Read the model definition and answer for the solid it produces. Units are mm, in the model's axes. A direction names the side the tool comes from. Give positions to 0.01 mm unless a question says otherwise; leave off trailing zeros. Write each loop counter-clockwise with the first axis right and the second up, starting at its lowest first coordinate (ties: lowest second). Pieces come first, ordered by that corner, then holes. Notation, with made-up numbers: (-1.5, 11) -> (53.5, 11) arc R18 ccw to (53.5, 27) -> close; hole circle Ø5 at (0, 32). An arc over 180 degrees is marked (long way). Use a Markdown table: item, result.
from build123d import *
from OCP.BRepFilletAPI import BRepFilletAPI_MakeChamfer

# Parameters (mm, degrees)
SKETCH1_W                = 120
SKETCH1_H                = 70
BOSS_EXTRUDE1_DEPTH      = 5
SKETCH4_W                = 10
SKETCH4_H                = 10
BOSS_EXTRUDE2_DEPTH      = 30
SKETCH5_W                = 10
SKETCH5_H                = 5
CUT_EXTRUDE2_DEPTH       = 10
SKETCH8_W                = 10
SKETCH8_H                = 7
BOSS_EXTRUDE5_DEPTH      = 4
M3_CLEARANCE_HOLE2_D     = 3.4
M3_CLEARANCE_HOLE2_DEPTH = 65
M3_CLEARANCE_HOLE2_TIP   = 1.021463052
SKETCH12_W               = 65.5
SKETCH12_H               = 70
BOSS_EXTRUDE6_DEPTH      = 5
BOSS_EXTRUDE7_DEPTH      = 35
M3_CLEARANCE_HOLE3_D     = 3.4
M3_CLEARANCE_HOLE3_DEPTH = 65
M3_CLEARANCE_HOLE3_TIP   = 1.021463052
SKETCH24_W               = 10
SKETCH24_H               = 50
BOSS_EXTRUDE10_DEPTH     = 10
SKETCH16_W               = 10
SKETCH16_H               = 22
CUT_EXTRUDE5_DEPTH       = 133.665933834
SKETCH22_R               = 1.7
CUT_EXTRUDE7_DEPTH       = 20
CHAMFER2_SIZE            = 10
CHAMFER2_SIZE_2          = 14
SKETCH25_W               = 5.49
SKETCH25_H               = 3
CUT_EXTRUDE8_DEPTH       = 8
CUT_EXTRUDE9_START       = -20
SKETCH26_R               = 1.7
CUT_EXTRUDE9_DEPTH       = 20
CUT_EXTRUDE11_DEPTH      = 10
LPATTERN1_COUNT          = 2
LPATTERN1_PITCH          = 110
SKETCH29_W               = 10
SKETCH29_H               = 4.75
BOSS_EXTRUDE11_DEPTH     = 15
SKETCH31_R               = 1.7
CUT_EXTRUDE13_DEPTH      = 153.152062096


with BuildPart() as part:
    # Sketch1 → Boss-Extrude1 (new body)
    with BuildSketch(Plane(origin=(0, 0, 0), x_dir=(1, 0, 0), z_dir=(0, 1, 0))):
        Rectangle(SKETCH1_W, SKETCH1_H)
    extrude(amount=BOSS_EXTRUDE1_DEPTH)

    # Sketch4 → Boss-Extrude2 (add)
    with BuildSketch(Plane(origin=(0, 5, 0), x_dir=(1, 0, 0), z_dir=(0, 1, 0))):
        with Locations((-55, -30)):
            Rectangle(SKETCH4_W, SKETCH4_H)
        with Locations((-55, 30)):
            Rectangle(SKETCH4_W, SKETCH4_H)
        with Locations((55, -30)):
            Rectangle(SKETCH4_W, SKETCH4_H)
        with Locations((55, 30)):
            Rectangle(SKETCH4_W, SKETCH4_H)
    extrude(amount=BOSS_EXTRUDE2_DEPTH)

    # Sketch5 → Cut-Extrude2 (cut)
    with BuildSketch(Plane.XZ):
        with Locations((-55, -27.5)):
            Rectangle(SKETCH5_W, SKETCH5_H)
        with Locations((-55, 27.5)):
            Rectangle(SKETCH5_W, SKETCH5_H)
        with Locations((55, 27.5)):
            Rectangle(SKETCH5_W, SKETCH5_H)
        with Locations((55, -27.5)):
            Rectangle(SKETCH5_W, SKETCH5_H)
    extrude(amount=-CUT_EXTRUDE2_DEPTH, mode=Mode.SUBTRACT)

    # Sketch8 → Boss-Extrude5 (add)
    with BuildSketch(Plane(origin=(0, 5, 0), x_dir=(1, 0, 0), z_dir=(0, 1, 0))):
        with Locations((-45, 31.5)):
            Rectangle(SKETCH8_W, SKETCH8_H)
        with Locations((-45, -31.5)):
            Rectangle(SKETCH8_W, SKETCH8_H)
        with Locations((45, -31.5)):
            Rectangle(SKETCH8_W, SKETCH8_H)
        with Locations((45, 31.5)):
            Rectangle(SKETCH8_W, SKETCH8_H)
    extrude(amount=BOSS_EXTRUDE5_DEPTH)

    # M3 Clearance Hole2
    with Locations(Plane(origin=(0, 9, 0), x_dir=(1, 0, 0), z_dir=(0, 1, 0))):
        with Locations((-43.5, -31.5), (-43.5, 31.5), (43.5, 31.5), (43.5, -31.5)):
            Hole(M3_CLEARANCE_HOLE2_D / 2, depth=M3_CLEARANCE_HOLE2_DEPTH)
            with Locations((0, 0, -(M3_CLEARANCE_HOLE2_DEPTH + M3_CLEARANCE_HOLE2_TIP / 2))):  # 118° drill point
                Cone(0, M3_CLEARANCE_HOLE2_D / 2, M3_CLEARANCE_HOLE2_TIP, mode=Mode.SUBTRACT)

    # Sketch12 → Boss-Extrude6 (add)
    with BuildSketch(Plane.XZ):
        with Locations((92.75, 0)):
            Rectangle(SKETCH12_W, SKETCH12_H)
    extrude(amount=-BOSS_EXTRUDE6_DEPTH)

    # Sketch13 → Boss-Extrude7 (add)
    with BuildSketch(Plane(origin=(0, 5, 0), x_dir=(1, 0, 0), z_dir=(0, 1, 0))):
        Polygon((60, 35), (125.5, 35), (125.5, -35), (60, -35), (60, -30.5), (121, -30.5), (121, 30.5), (60, 30.5), align=None)
    extrude(amount=BOSS_EXTRUDE7_DEPTH)

    # M3 Clearance Hole3
    with Locations(Plane(origin=(0, 5, 0), x_dir=(1, 0, 0), z_dir=(0, 1, 0))):
        with Locations((117, -26.5), (117, 26.5), (64, 26.5), (64, -26.5)):
            Hole(M3_CLEARANCE_HOLE3_D / 2, depth=M3_CLEARANCE_HOLE3_DEPTH)
            with Locations((0, 0, -(M3_CLEARANCE_HOLE3_DEPTH + M3_CLEARANCE_HOLE3_TIP / 2))):  # 118° drill point
                Cone(0, M3_CLEARANCE_HOLE3_D / 2, M3_CLEARANCE_HOLE3_TIP, mode=Mode.SUBTRACT)

    # Sketch24 → Boss-Extrude10 (add)
    with BuildSketch(Plane(origin=(0, 5, 0), x_dir=(1, 0, 0), z_dir=(0, 1, 0))):
        with Locations((-55, 0)):
            Rectangle(SKETCH24_W, SKETCH24_H)
        with Locations((55, 0)):
            Rectangle(SKETCH24_W, SKETCH24_H)
    extrude(amount=BOSS_EXTRUDE10_DEPTH)

    # Sketch16 → Cut-Extrude5 (cut, through all)
    with BuildSketch(Plane(origin=(0, 15, 0), x_dir=(1, 0, 0), z_dir=(0, 1, 0))):
        with Locations((55, 0)):
            Rectangle(SKETCH16_W, SKETCH16_H)
    extrude(amount=-CUT_EXTRUDE5_DEPTH, mode=Mode.SUBTRACT)

    # Sketch22 → Cut-Extrude7 (cut)
    with BuildSketch(Plane.XY.offset(35)):
        with Locations((-55, 5)):
            Circle(SKETCH22_R)
        with Locations((55, 5)):
            Circle(SKETCH22_R)
    extrude(amount=-CUT_EXTRUDE7_DEPTH, mode=Mode.SUBTRACT)

    # Chamfer2
    chamfer2_edges_1 = [part.edges().sort_by_distance(p)[0] for p in [
        (55, 15, 11),
    ]]
    chamfer2_side_1 = [part.faces().sort_by_distance(p)[0] for p in [
        (55, 14.8, 11),
    ]]
    chamfer2_edges_2 = [part.edges().sort_by_distance(p)[0] for p in [
        (55, 15, -11),
    ]]
    chamfer2_side_2 = [part.faces().sort_by_distance(p)[0] for p in [
        (55, 14.8, -11),
    ]]
    chamfer2 = BRepFilletAPI_MakeChamfer(part.part.solid().wrapped)
    for e in chamfer2_edges_1:
        chamfer2.Add(CHAMFER2_SIZE - 0.0001, CHAMFER2_SIZE_2 - 0.0001, e.wrapped, chamfer2_side_1[0].wrapped)
    for e in chamfer2_edges_2:
        chamfer2.Add(CHAMFER2_SIZE - 0.0001, CHAMFER2_SIZE_2 - 0.0001, e.wrapped, chamfer2_side_2[0].wrapped)
    add(Compound.cast(chamfer2.Shape()), mode=Mode.REPLACE)  # a hair under: the kernel refuses the full size

    # Sketch25 → Cut-Extrude8 (cut)
    with BuildSketch(Plane.XZ):
        with Locations((-55, -18.5)):
            Rectangle(SKETCH25_W, SKETCH25_H)
        with Locations((55, -18.5)):
            Rectangle(SKETCH25_W, SKETCH25_H)
        with Locations((55, 18.5)):
            Rectangle(SKETCH25_W, SKETCH25_H)
        with Locations((-55, 18.5)):
            Rectangle(SKETCH25_W, SKETCH25_H)
    extrude(amount=-CUT_EXTRUDE8_DEPTH, mode=Mode.SUBTRACT)

    # Sketch26 → Cut-Extrude9 (cut)
    with BuildSketch(Plane(origin=(0, 0, -35), x_dir=(-1, 0, 0), z_dir=(0, 0, -1)).offset(CUT_EXTRUDE9_START)):
        with Locations(Location((-55, 5, 0), (0, 0, 180))):
            Circle(SKETCH26_R)
        with Locations(Location((55, 5, 0), (0, 0, 180))):
            Circle(SKETCH26_R)
    extrude(amount=CUT_EXTRUDE9_DEPTH, mode=Mode.SUBTRACT)

    # Sketch28 → Cut-Extrude11 (cut)
    with BuildSketch(Plane.ZY.offset(60)):
        Polygon((-25, 10), (-23, 0), (-25, 0), align=None)
        Polygon((25, 10), (23, 0), (25, 0), align=None)
    cut_extrude11 = extrude(amount=-CUT_EXTRUDE11_DEPTH, mode=Mode.SUBTRACT)

    # LPattern1: Cut-Extrude11 ×2
    with Locations(*[(i * LPATTERN1_PITCH, 0, 0) for i in range(1, LPATTERN1_COUNT)]):
        add(cut_extrude11, mode=Mode.SUBTRACT)

    # Sketch29 → Boss-Extrude11 (add)
    with BuildSketch(Plane(origin=(0, 35, 0), x_dir=(1, 0, 0), z_dir=(0, 1, 0))):
        with Locations((55, 32.625)):
            Rectangle(SKETCH29_W, SKETCH29_H)
        with Locations((55, -32.625)):
            Rectangle(SKETCH29_W, SKETCH29_H)
        with Locations((-55, 32.625)):
            Rectangle(SKETCH29_W, SKETCH29_H)
        with Locations((-55, -32.625)):
            Rectangle(SKETCH29_W, SKETCH29_H)
    extrude(amount=BOSS_EXTRUDE11_DEPTH)

    # Sketch31 → Cut-Extrude13 (cut, through all)
    with BuildSketch(Plane(origin=(0, 0, -35), x_dir=(-1, 0, 0), z_dir=(0, 0, -1))):
        with Locations((-55, 45)):
            Circle(SKETCH31_R)
        with Locations((55, 45)):
            Circle(SKETCH31_R)
    extrude(amount=-CUT_EXTRUDE13_DEPTH, mode=Mode.SUBTRACT)


solid = part.part
Item 1: A cutting plane is placed at D-D (x = 96.5). Give the vertices of the cut face in (y, z), then the cut area to 3 significant figures.
Return value:
| item | result |
|---|---|
| outline | (0, -35) -> (40, -35) -> (40, -30.5) -> (5, -30.5) -> (5, 30.5) -> (40, 30.5) -> (40, 35) -> (0, 35) -> close |
| area | 665 mm^2 |
Item 2: Each of these flat-tipped pins is pushed along its axis until it touches: P1, Ø1.6, axis at x = 56, y = 5.5, coming from the +Z side; P2, Ø10, axis at x = 14.5, z = -21, coming from the +Y side; P3, Ø1.6, axis at x = -56, z = 27.5, coming from the +Y side; P4, Ø7.5, axis at x = 45, z = 32.5, coming from the +Y side. Where does it stop, or does it pass through?
Return value:
| item | result |
|---|---|
| P1 | z = 35 |
| P2 | y = 5 |
| P3 | y = 35 |
| P4 | y = 9 |
Item 3: Straight lines are drawn through the part: line 1 along X through (y, z) = (13, -29); line 2 along Y through (x, z) = (-55, -32.15); line 3 along Z through (x, y) = (110.5, 33.5). For each, find the intervals that lie inside material, in ascending order. Write a range as [from, to].
Return value:
| item | result |
|---|---|
| line 1 | [-60, -50], [50, 60], [121, 125.5] |
| line 2 | [0, 3.3], [6.7, 43.3], [46.7, 50] |
| line 3 | [-35, -30.5], [30.5, 35] |
Item 4: A cutting plane is placed at A-A (x = 43.5). Give the vertices of the cut face in (y, z), then the cut area to 3 significant figures.
Return value:
| item | result |
|---|---|
| outline | (0, -35) -> (9, -35) -> (9, -33.2) -> (0, -33.2) -> close; (0, -29.8) -> (9, -29.8) -> (9, -28) -> (5, -28) -> (5, 28) -> (9, 28) -> (9, 29.8) -> (0, 29.8) -> close; (0, 33.2) -> (9, 33.2) -> (9, 35) -> (0, 35) -> close |
| area | 345 mm^2 |
Item 5: A cutting plane is placed at C-C (y = 23). Give the vertices of the cut face in (x, z).
Return value:
| item | result |
|---|---|
| outline | (-60, -35) -> (-50, -35) -> (-50, -25) -> (-60, -25) -> close; (-60, 25) -> (-50, 25) -> (-50, 35) -> (-60, 35) -> close; (50, -35) -> (125.5, -35) -> (125.5, 35) -> (50, 35) -> (50, 25) -> (60, 25) -> (60, 30.5) -> (121, 30.5) -> (121, -30.5) -> (60, -30.5) -> (60, -25) -> (50, -25) -> close |
Item 6: A tool of negligible diameter and unlimited length cuts with its end or side. For faces 1 (the face through (55, 25, 25)), 2 (the face through (122, 40, 2)), 3 (the face through (55, 3, 11)), 4 (the face through (-56.7, 5.07, 32.53)), from which of +Z, -Z, +X, -X, +Y, -Y can it reach the whole face along a straight path? Write none if from no direction.
Return value:
| item | result |
|---|---|
| face 1 | -X, +Y |
| face 2 | +Z, -Z, +X, +Y |
| face 3 | +Y, -Y |
| face 4 | +Z |
Item 7: For a pull along Y with two mould halves and no side action, classify faces 5 (the face through (-45, 7, -28)), 6 (the face through (-55, 5, 15)), 7 (the face through (53, 5, 24)) as +Y half, -Y half, draft (parallel to the pull), parting line (faces both ways), or undercut.
Return value:
| item | result |
|---|---|
| face 5 | draft |
| face 6 | undercut |
| face 7 | -Y half |
Item 8: A cutting plane is placed at B-B (z = -7). Give the vertices of the cut face in (x, y).
Return value:
| item | result |
|---|---|
| outline | (-60, 0) -> (50, 0) -> (50, 5) -> (-50, 5) -> (-50, 15) -> (-60, 15) -> close; (60, 0) -> (125.5, 0) -> (125.5, 40) -> (121, 40) -> (121, 5) -> (60, 5) -> close |
